Could you check a few things on this model? Use its own coordinates, in mm. Give positions to 0.01 mm unless a question says otherwise; leave off trailing zeros. Order: outer loops, then holes, each group sorted by start corner. A loop starts at its lowest first (then second) coordinate and runs counter-clockwise, first axis right, second up.
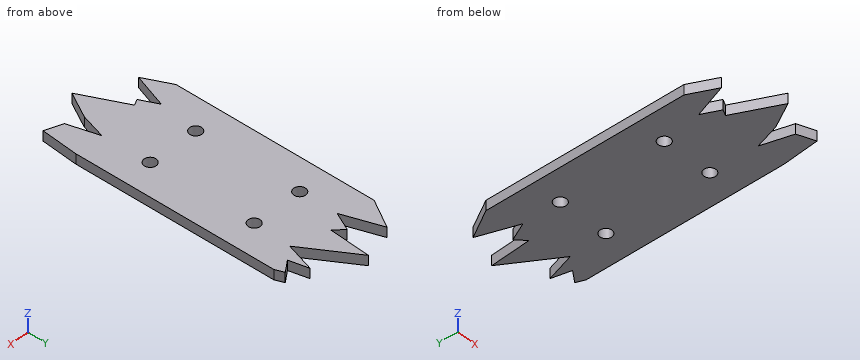
from build123d import *

# Parameters (mm, degrees)
F1_DEPTH = 10
F2_R     = 6
F3_DEPTH = 10.001


# Not quite as in the source:
# - a pattern or mirror of a feature is missing from the dataset's text; its kind, count and spacing are read off the source's solid


with BuildPart() as f1:
    # F0 (on Top) → F1 (new body)
    with BuildSketch(Plane.XY):
        Polygon((-55, 100), (-55, -100), (-42.3276498914, -126.1771321297), (-30.6749343872, -92.5011336803), (-22.4767297883, -109.4360733855), (-16.331512481, -106.4611735826), (4.8077032396, -150.1282154724), (18.9439784735, -124.5355084538), (26.3201091439, -100), (34.8079055548, -130.0195604563), (51.677390933, -136.1848264933), (55, -100), (55, 100), (51.677390933, 108.4323301911), (40.0880090892, 100), (35.7317700982, 118.9388260245), (26.9271209836, 90.1910439134), (-4.7420188785, 140.4679864645), (-7.6231127605, 100), (-16.331512481, 108.4323301911), (-25.1079257578, 90.1910439134), (-38.313575089, 128.3779740334), align=None)
    extrude(amount=F1_DEPTH)

    # F2 (on face) → F3 (cut, through all)
    with BuildSketch(Plane.XY.offset(10)):
        with Locations((-25, 52.5)):
            Circle(F2_R)
    f3 = extrude(amount=-F3_DEPTH, mode=Mode.SUBTRACT)

    # F3_copies: F3 across plane
    add(f3.mirror(Plane(origin=(0, 0, 0), x_dir=(0, 0, -1), z_dir=(0, -1, 0))), mode=Mode.SUBTRACT)

    # F3_copies1: F3 across plane
    add(f3.mirror(Plane(origin=(0, 0, 0), x_dir=(0, 0, 1), z_dir=(1, 0, 0))), mode=Mode.SUBTRACT)

    # F3_copies2: F3 across plane
    add(f3.mirror(Plane(origin=(0, 0, 0), x_dir=(-0.9028605188, -0.4299335804, 0), z_dir=(0.4299335804, -0.9028605188, 0))), mode=Mode.SUBTRACT)


solid = f1.part
Item 1: Imagine slicing it at C-C on x = -1. List the corners of the cut face in (y, z) for me.
Findings:
outline: (-138.13, 0) - (134.53, 0) - (134.53, 10) - (-138.13, 10) - close
Item 2: For pin 1 (6 mm diameter, centred on x = -19.5, z = 8, fed in from -Y); pin 2 (4 mm diameter, centred on x = -16.5, z = 3.5, fed in from +Y); pin 3 (1 mm diameter, centred on x = -24, z = 3, fed in from -Y), each with a flat end and sliding along its axis, tell me the tip position at first contact or that it passes through.
Findings:
pin 1: stops at y = -109.44
pin 2: stops at y = 108.43
pin 3: stops at y = -107.32
Item 3: Imagine slicing it at B-B on z = 1.5. List the corners of the cut face in (x, y) for me.
Findings:
outline: (-55, -100) - (-42.33, -126.18) - (-30.67, -92.5) - (-22.48, -109.44) - (-16.33, -106.46) - (4.81, -150.13) - (18.94, -124.54) - (26.32, -100) - (34.81, -130.02) - (51.68, -136.18) - (55, -100) - (55, 100) - (51.68, 108.43) - (40.09, 100) - (35.73, 118.94) - (26.93, 90.19) - (-4.74, 140.47) - (-7.62, 100) - (-16.33, 108.43) - (-25.11, 90.19) - (-38.31, 128.38) - (-55, 100) - close; hole circle Ø12 at (-25, -52.5); hole circle Ø12 at (-25, 52.5); hole circle Ø12 at (25, -52.5); hole circle Ø12 at (25, 52.5)
Item 4: Imagine slicing it at A-A on y = -52.5. List the corners of the cut face in (x, z) for me.
Findings:
outline: (-55, 0) - (-31, 0) - (-31, 10) - (-55, 10) - close; (-19, 0) - (19, 0) - (19, 10) - (-19, 10) - close; (31, 0) - (55, 0) - (55, 10) - (31, 10) - close
Item 5: Please list where these lines run through material, in increasing order: line 1 along X through (y, z) = (-52.5, 7); line 2 along X through (y, z) = (-112.5, 3.5); line 3 along Y through (x, z) = (-25, 6.75).
Findings:
line 1: x = -55 to -31, -19 to 19, 31 to 55
line 2: x = -48.95 to -37.6, -13.41 to 22.56, 29.85 to 53.85
line 3: y = -104.22 to -58.5, -46.5 to 46.5, 58.5 to 90.42
